from build123d import *

# Parameters (mm, degrees)
F1_DEPTH  = 14.986
F2_R      = 0.508
F3_DEPTH  = 8.382
F4_R      = 0.635
F5_DEPTH  = 5.08
F6_R      = 1.9685
F7_DEPTH  = 0.635
F8_R      = 1.905
F9_DEPTH  = 1.143
F11_DEPTH = 1.524


with BuildPart() as f1:
    # F0 (on Front) → F1 (new body)
    with BuildSketch(Plane.XZ):
        with BuildLine():
            Line((4.0005, -3.175), (4.0005, 3.175))
            ThreePointArc((4.0005, 3.175), (0, 4.953), (-4.0005, 3.175))
            Line((-4.0005, 3.175), (-4.0005, -3.175))
            ThreePointArc((-4.0005, -3.175), (0, -4.953), (4.0005, -3.175))
        make_face()
    extrude(amount=-F1_DEPTH)

    # F2 (on face) → F3 (join)
    with BuildSketch(Plane.XZ):
        Circle(F2_R)
    extrude(amount=F3_DEPTH)

    # F4 (on face) → F5 (cut)
    with BuildSketch(Plane.XZ):
        with Locations((0, 3.4925)):
            Circle(F4_R)
        with Locations((0, -3.4925)):
            Circle(F4_R)
    extrude(amount=-F5_DEPTH, mode=Mode.SUBTRACT)

    # F6 (on face) → F7 (join)
    with BuildSketch(Plane.XZ):
        Circle(F6_R)
    extrude(amount=F7_DEPTH)

    # F8 (on face) → F9 (join)
    with BuildSketch(Plane(origin=(0, 14.986, 0), x_dir=(-1, 0, 0), z_dir=(0, 1, 0))):
        Circle(F8_R)
    extrude(amount=F9_DEPTH)

    # F10 (on face) → F11 (join)
    with BuildSketch(Plane(origin=(0, 14.986, 0), x_dir=(-1, 0, 0), z_dir=(0, 1, 0))):
        Polygon((-2.028809, -2.891869), (-2.13069, -3.124541), (-0.850995, -3.684889), (-0.749114, -3.452217), align=None)
        Polygon((0.850995, 3.684889), (0.749114, 3.452217), (2.028809, 2.891869), (2.13069, 3.124541), align=None)
    extrude(amount=F11_DEPTH)


solid = f1.part
Geometry check sheet. Reference: the model listing, model coordinates, mm. A direction names the side the tool comes from. Give positions to 0.01 mm unless a question says otherwise; leave off trailing zeros. Write each loop counter-clockwise with the first axis right and the second up, starting at its lowest first coordinate (ties: lowest second). Pieces come first, ordered by that corner, then holes.
1) Thickness scan on line 1 (X direction, y = 2.5, z = 3.5); line 2 (Z direction, x = 0.25, y = 3); line 3 (Y direction, x = -3, z = 1.5). Record the ranges inside material, lowest first.
Values follow:
line 1: x = -3.68 to -0.63, 0.63 to 3.68
line 2: z = -4.95 to -4.08, -2.91 to 2.91, 4.08 to 4.95
line 3: y = 0 to 14.99
2) Cross-section at B-B (x = 0). Record the boundary of the cut face in (y, z) (1 decimal), plus the area to 3 significant figures.
Values follow:
outline: (-8.4, -0.5) - (-0.6, -0.5) - (-0.6, -2) - (0, -2) - (0, -2.9) - (5.1, -2.9) - (5.1, -4.1) - (0, -4.1) - (0, -5) - (15, -5) - (15, -1.9) - (16.1, -1.9) - (16.1, 1.9) - (15, 1.9) - (15, 5) - (0, 5) - (0, 4.1) - (5.1, 4.1) - (5.1, 2.9) - (0, 2.9) - (0, 2) - (-0.6, 2) - (-0.6, 0.5) - (-8.4, 0.5) - close
area: 150 mm2
3) Cross-section at A-A (z = 1.5). Record the boundary of the cut face in (x, y) (1 decimal), plus the area to 3 significant figures.
Values follow:
outline: (-4, 0) - (-1.3, 0) - (-1.3, -0.6) - (1.3, -0.6) - (1.3, 0) - (4, 0) - (4, 15) - (1.2, 15) - (1.2, 16.1) - (-1.2, 16.1) - (-1.2, 15) - (-4, 15) - close
area: 124 mm2
4) Set-up check for faces 4 (the face through (0, 5.08, 3.5)), 5 (the face through (-1.5, 15.7, 3.4)), 6 (the face through (1.5, 15.7, -3.4)), 7 (the face through (1.38, 15.737, -3.176)), 8 (the face through (-2, 14.986, 1)): record each of +Z, -Z, +X, -X, +Y, -Y from which the full face is reachable in a straight line by a thin tool's end or side.
Values follow:
face 4: -Y
face 5: +Z, -X, +Y
face 6: -Z, +X, +Y
face 7: -X, +Y
face 8: +Y
5) Cross-section at D-D (y = 3.25). Record the boundary of the cut face in (x, z) (1 decimal).
Values follow:
outline: (-4, -3.2) arc R5.4 ccw to (4, -3.2) - (4, 3.2) arc R5.4 ccw to (-4, 3.2) - close; hole circle Ø1.3 at (0, -3.5); hole circle Ø1.3 at (0, 3.5)
6) Cross-section at C-C (y = 8.25). Record the boundary of the cut face in (x, z) (1 decimal), plus the area to 3 significant figures.
Values follow:
outline: (-4, -3.2) arc R5.4 ccw to (4, -3.2) - (4, 3.2) arc R5.4 ccw to (-4, 3.2) - close
area: 70.5 mm2
7) Go/stop test with flat-tipped pins: pin 1 Ø2.5 at (x, z) = (0, 0.5) entering from +Y; pin 2 Ø0.8 at (x, z) = (0, 3.49) entering from +Y; pin 3 Ø0.6 at (x, z) = (0, -4) entering from -Y; pin 4 Ø4.5 at (x, z) = (-1, 0) entering from -Y. Record where each tip stops, or that it passes through.
Values follow:
pin 1: stops at y = 16.13
pin 2: stops at y = 14.99
pin 3: stops at y = 0
pin 4: stops at y = -8.38
8) Release check for a two-part mould opening along X. For faces 1 (the face through (0, 5.08, -3.5)), 2 (the face through (-2, 0, 1)), 3 (the face through (4, 7, 0)) record: released by +X, released by -X, zero draft, split by the parting line, or undercut.
Values follow:
face 1: undercut
face 2: zero draft
face 3: released by +X
